Autodesk Inventor part; units mm, degrees
ref_plane "Work Plane1" through (0, 196.85, 0) normal (0, 1, 0) x (-1, 0, 0)
ref_plane "YZ Plane" through (0, 0, 0) normal (1, 0, 0) x (0, 1, 0)
ref_plane "XY Plane" through (0, 0, 0) normal (0, 0, 1) x (1, 0, 0)
sketch "Sketch1" plane through (0, 0, 0) normal (1, 0, 0) x (0, 1, 0)
  arc A0 (-152.4, 0) -> (152.4, 0) centre (0, 0) ccw
  arc A1 (-149.35, 0) -> (149.35, 0) centre (0, 0) ccw
  line L0 (152.4, 0) -> (149.35, 0)
  line L1 (-149.35, 0) -> (-152.4, 0)
  line L2 (-213.36, 0) -> (213.36, 0)
  dimension "d0" = 152.4
  dimension "d2" = 149.35
revolve "Revolution1" add sketch "Sketch1" angle 360 about axis through (0, -10, 0) along (0, 1, 0) contours L1 A1 L0 A0
sketch "Sketch2" plane through (0, 0, 0) normal (1, 0, 0) x (0, 1, 0)
  circle A0 centre (0, 0) radius 98.5
  dimension "d4" = 197
extrude "Extrusion1" cut sketch "Sketch2" along normal through all both and the other way through all
sketch "Sketch3" plane through (0, 0, 0) normal (0, 1, 0) x (-1, 0, 0)
  circle A0 centre (0, 0) radius 98.5
  dimension "d7" = 197
extrude "Extrusion2" cut sketch "Sketch3" along normal through all both and the other way through all
ref_plane "Work Plane1" through (0, 196.85, 0) normal (0, 1, 0) x (-1, 0, 0)
sketch "Sketch4" plane through (0, 196.85, 0) normal (0, 1, 0) x (-1, 0, 0)
  circle A0 centre (0, 0) radius 101.6
  circle A1 centre (0, 0) radius 98.5
  circle A2 centre (0, 0) radius 98.5
  dimension "d11" = 203.2
  dimension "d12" = 197
extrude "Extrusion3" add sketch "Sketch4" against normal up to next
pattern_circular "Circular Pattern1" count 4 over 360 about axis through (0, 0, -10) along (0, 0, 1) of "Extrusion3"
properties part number "ISO_200_Cross_4way_Sphere"
The model under review builds one solid part; all positions refer to its coordinate system, in mm. A direction names the side the tool comes from. Give positions to 0.01 mm unless a question says otherwise; leave off trailing zeros. Order: outer loops, then holes, each group sorted by start corner. A loop starts at its lowest first (then second) coordinate and runs counter-clockwise, first axis right, second up. Notation, with made-up numbers: M 12.5,81 L 50.5,81 A16 ccw 50.5,92 Z; hole C 55,56.25 d4. An arc over 180 degrees is marked long. One line per question, with ' | ' between items. Start each with the question number.
1) Consider section A-A, the plane x = 0. Give the boundary of the cut face in (y, z).
2) Wall thickness on L1, parallel to Z at x = -142, y = 0; L2, parallel to Z at x = -30.5, y = -88; L3, parallel to Y at x = -139, z = 17.5: over which ranges is each line inside the solid? List them lowest first. Write a range as from..to.
3) Consider section D-D, the plane y = -170.5. Give the boundary of the cut face in (x, z), then the cut area to 3 significant figures.
4) Consider section B-B, the plane z = 0. State how many separate pieces and enclosed holes the cut face has, then the cut area to 3 significant figures.
5) Clearance check with flat-ended pins moving along their axes: P1, Ø3, axis at x = 154.5, z = 67, coming from the -Y side; P2, Ø3, axis at x = -92, y = -148.5, coming from the +Z side; P3, Ø12, axis at x = -24, y = 53, coming from the +Z side. State where each tip first meets the part, or that it passes through.
6) For faces 1 (the face through (155.804, -22.025, -99.184)), 2 (the face through (-22.025, -155.804, -99.184)), 3 (the face through (22.025, 155.804, -99.184)), list the 3-axis set-ups (+Z, -Z, +X, -X, +Y, -Y) from which the entire face can be reached by the end or side of a thin tool; tool diameter is ignored.
7) Mouldability with a two-part tool opening along X and no side actions: class faces 4 (the face through (196.85, -53.2, 83.3)), 5 (the face through (53.2, 196.85, 83.3)), 6 (the face through (-93.95, 153.96, -29.59)) as pulls with the +X half, pulls with the -X half, needs draft (parallel to the pull), parting line crosses it, or undercut.
Found:
1) outline: M -196.85,-101.6 L -113.59,-101.6 A152.4 ccw 113.59,-101.6 L 196.85,-101.6 L 196.85,-98.5 L 112.26,-98.5 A149.35 cw -112.26,-98.5 L -196.85,-98.5 Z; M -196.85,98.5 L -112.26,98.5 A149.35 cw 112.26,98.5 L 196.85,98.5 L 196.85,101.6 L 113.59,101.6 A152.4 ccw -113.59,101.6 L -196.85,101.6 Z
2) L1: z = -101.6..-98.5, 98.5..101.6 | L2: z = -120.63..-116.75, 116.75..120.63 | L3: y = -100.08..-96.93, 96.93..100.08
3) outline: C 0,0 d203.2; hole C 0,0 d197 | area: 1,950 mm²
4) separate pieces: 4 | enclosed holes: 0 | area: 2,300 mm²
5) P1: stops at y = -77.67 | P2: stops at z = 46.18 | P3: stops at z = 143.19
6) face 1: +X | face 2: -Y | face 3: +Y
7) face 4: pulls with the +X half | face 5: needs draft | face 6: undercut
